Work out the finished part from the listing and answer in its coordinate system (mm). Face numbers are marked on the shaded views. A direction names the side the tool comes from. Round coordinates to 2 decimals unless told otherwise and drop trailing zeros. Order: outer loops, then holes, each group sorted by start corner. A loop starts at its lowest first (then second) coordinate and runs counter-clockwise, first axis right, second up. Notation, with made-up numbers: (44, 2.25) - (79, 2.25) arc R21 cw to (79, 36.25) - close; hole circle Ø8 at (48.25, 25.25). An arc over 180 degrees is marked (long way). Put each result on its own line as item: value.
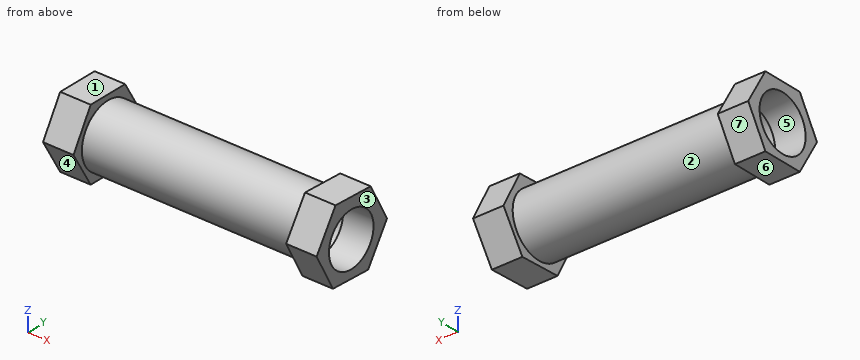
```python
from build123d import *

# Parameters (mm, degrees)
SKETCH1_R            = 50.800375113
SKETCH1_R_2          = 47.812951641
BOSS_EXTRUDE2_DEPTH  = 350
BOSS_EXTRUDE5_DEPTH  = 50
BOSS_EXTRUDE11_DEPTH = 50
SKETCH6_R            = 44.996318031
CUT_EXTRUDE2_DEPTH   = 50
SKETCH7_R            = 43.517898498
CUT_EXTRUDE3_DEPTH   = 50


with BuildPart() as part:
    # Sketch1 → Boss-Extrude2 (new body)
    with BuildSketch(Plane(origin=(0, 0, 0), x_dir=(0, 0, -1), z_dir=(1, 0, 0))):
        with Locations((1.289702318, 0)):
            Circle(SKETCH1_R)
        with Locations((1.289702318, 0)):
            Circle(SKETCH1_R_2, mode=Mode.SUBTRACT)
    extrude(amount=BOSS_EXTRUDE2_DEPTH)

    # Sketch3 → Boss-Extrude5 (add)
    with BuildSketch(Plane(origin=(350, 0, 0), x_dir=(0, 0, -1), z_dir=(1, 0, 0))):
        Polygon((58.055626726, -36.855405481), (60.945530776, 31.849944836), (2.88990405, 68.705350317), (-58.055626726, 36.855405481), (-60.945530776, -31.849944836), (-2.88990405, -68.705350317), align=None)
        Polygon((29.411876605, -18.99044871), (30.315925302, 11.383738416), (4.46313198, 27.353761118), (-22.293710039, 12.949596693), (-23.197758737, -17.424590433), (2.655034585, -33.394613135), align=None, mode=Mode.SUBTRACT)
    extrude(amount=BOSS_EXTRUDE5_DEPTH)

    # Sketch5 → Boss-Extrude11 (add)
    with BuildSketch(Plane.ZY):
        Polygon((0, -67.161353017), (58.163437865, -33.580676508), (58.163437865, 33.580676508), (0, 67.161353017), (-58.163437865, 33.580676508), (-58.163437865, -33.580676508), align=None)
    extrude(amount=BOSS_EXTRUDE11_DEPTH)

    # Sketch6 → Cut-Extrude2 (cut)
    with BuildSketch(Plane(origin=(0, 0, 0), x_dir=(0, 0, -1), z_dir=(1, 0, 0))):
        with Locations((2.167278034, 0)):
            Circle(SKETCH6_R)
    extrude(amount=-CUT_EXTRUDE2_DEPTH, mode=Mode.SUBTRACT)

    # Sketch7 → Cut-Extrude3 (cut)
    with BuildSketch(Plane.ZY.offset(-350)):
        with Locations((-2.231478452, -1.09442532)):
            Circle(SKETCH7_R)
    extrude(amount=-CUT_EXTRUDE3_DEPTH, mode=Mode.SUBTRACT)


solid = part.part
```
1) A cutting plane is placed at C-C on z = -25.5. Write down the section's boundary in (x, y), then the cut area to 3 significant figures.
Findings below:
outline: (-50, -52.44) - (0, -52.44) - (0, -44.66) - (350, -44.66) - (350, -53.87) - (400, -53.87) - (400, -37.87) - (350, -37.87) - (350, -41.23) - (0, -41.23) - (0, -38.47) - (-50, -38.47) - close; (-50, 38.47) - (0, 38.47) - (0, 41.23) - (350, 41.23) - (350, 35.68) - (400, 35.68) - (400, 54.35) - (350, 54.35) - (350, 44.66) - (0, 44.66) - (0, 52.44) - (-50, 52.44) - close
area: 5,530 mm2
2) A cutting plane is placed at B-B on y = -21. Write down the section's boundary in (x, z).
Findings below:
outline: (-50, -58.16) - (0, -58.16) - (0, -47.55) - (350, -47.55) - (350, -58.72) - (400, -58.72) - (400, -40.93) - (350, -40.93) - (350, -44.24) - (0, -44.24) - (0, -41.96) - (-50, -41.96) - close; (-50, 37.63) - (0, 37.63) - (0, 41.66) - (350, 41.66) - (350, 36.47) - (400, 36.47) - (400, 60.49) - (350, 60.49) - (350, 44.97) - (0, 44.97) - (0, 58.16) - (-50, 58.16) - close
3) A cutting plane is placed at D-D on y = 59. Write down the section's boundary in (x, z), then the cut area to 3 significant figures.
Findings below:
outline: (-50, -14.14) - (0, -14.14) - (0, 14.14) - (-50, 14.14) - close; (350, -18.18) - (400, -18.18) - (400, 15.68) - (350, 15.68) - close
area: 3,110 mm2
4) For a pull along X with two mould halves and no side action, classify the marked faces 1, 2 and 3 as pulls with the +X half, pulls with the -X half, needs draft (parallel to the pull), parting line crosses it, or undercut.
Findings below:
face 1: needs draft
face 2: undercut
face 3: pulls with the +X half
5) For the marked faces 4, 5, 6 and 7, determine the directions among +Z, -Z, +X, -X, +Y, -Y from which every point of the face is accessible in a straight line to the end or side of a thin tool.
Findings below:
face 4: -Z, -X, -Y
face 5: -X
face 6: -Z, -X, +Y, -Y
face 7: -Z, -X, +Y
6) Straight lines are drawn through the part: L1, parallel to X at y = -39, z = -48; L2, parallel to Z at x = 94.5, y = -2; L3, parallel to Y at x = 170.5, z = -38. For each, find the intervals that lie inside material, in ascending order. Write a range as from..to.
Findings below:
L1: x = -50..0, 350..400
L2: z = -52.05..-49.06, 46.48..49.47
L3: y = -35.11..-30.63, 30.63..35.11
7) A cutting plane is placed at A-A on x = -5.5. Write down the section's boundary in (y, z).
Findings below:
outline: (-67.16, 0) - (-33.58, -58.16) - (33.58, -58.16) - (67.16, 0) - (33.58, 58.16) - (-33.58, 58.16) - close; hole circle Ø89.99 at (0, -2.17)
8) Given pin 1 Ø5 at (x, y) = (12, -46.5) entering from -Z; pin 2 Ø6 at (x, y) = (249, -54.5) entering from +Z; pin 3 Ø25 at (x, y) = (-31, 14.5) entering from -Z; pin 4 Ø1.5 at (x, y) = (97, -33) entering from -Z, each flat-ended and moving along its own axis, determine where each tip first touches the part or whether it passes through.
Findings below:
pin 1: stops at z = -26.68
pin 2: passes through
pin 3: stops at z = -58.16
pin 4: stops at z = -40.54
